The figure shows three views and two pictorial views of one solid part (mm, origin at its lowest corner). Answer the questions. Coordinates: 2 decimals unless noted, no trailing zeros. Loops run counter-clockwise (first coordinate to the right, second up) from the corner with the lowest first, then second, coordinate; pieces in that order, holes last. Notation, with made-up numbers: M -20,0 L -5,0 A26 cw -5,27 Z; hole C 35.25,-27 d11. An arc over 180 degrees is marked long. Write each question's results on one line, items separated by ' | '.
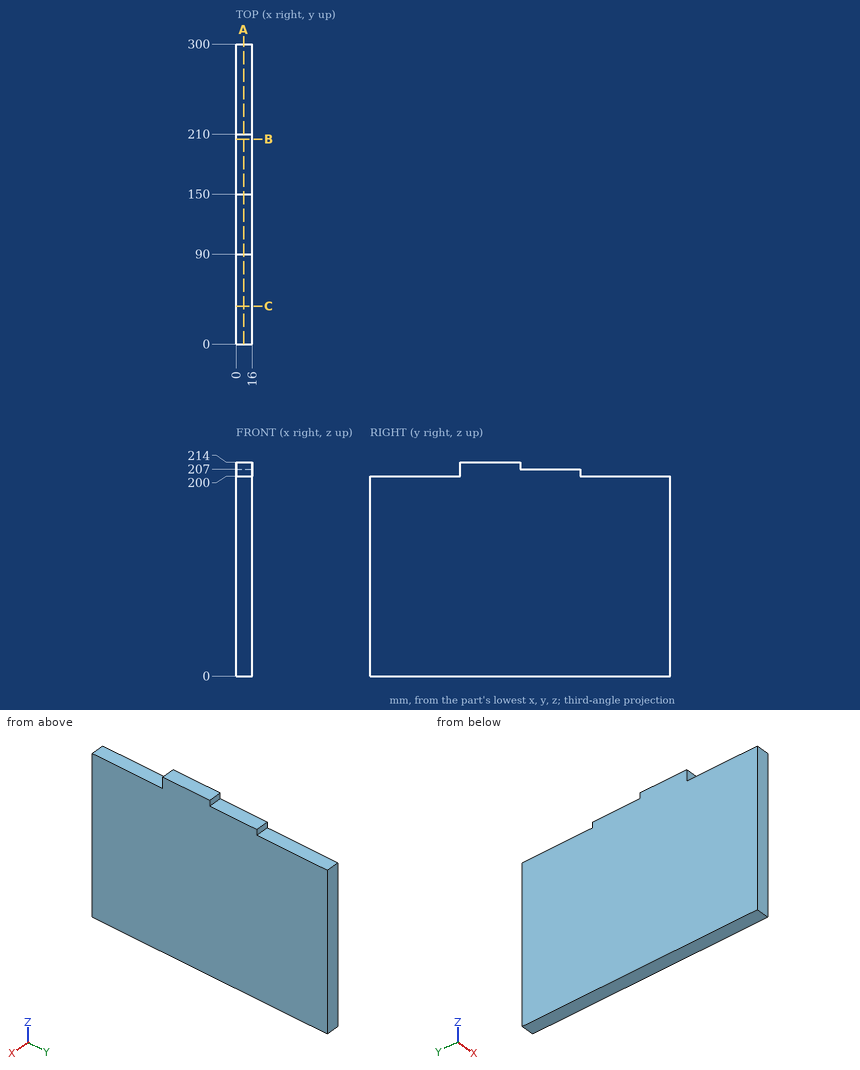
1) Straight lines are drawn through the part: probe 1 along Z at (x, y) = (7, 80.5); probe 2 along Z at (x, y) = (3.75, 168). For each, find the intervals that lie inside material, in ascending order. Write a range as [from, to].
Check result:
probe 1: [0, 200] | probe 2: [0, 207]
2) Find section C-C, the plane y = 38. Give the vertices of the cut face in (x, z), and give its area (3 significant figures).
Check result:
outline: M 0,0 L 16,0 L 16,200 L 0,200 Z | area: 3,200 mm^2
3) Find section B-B, the plane y = 205. Give the vertices of the cut face in (x, z), and give its area (3 significant figures).
Check result:
outline: M 0,0 L 16,0 L 16,207 L 0,207 Z | area: 3,310 mm^2
4) Given pin 1 Ø8 at (x, y) = (8.5, 189) entering from +Z; pin 2 Ø3.5 at (x, z) = (10, 204) entering from +Y; pin 3 Ø2 at (x, z) = (11.5, 210.5) entering from +Y, each flat-ended and moving along its own axis, determine where each tip first touches the part or whether it passes through.
Check result:
pin 1: z = 207 | pin 2: y = 210 | pin 3: y = 150
5) Find section A-A, the plane x = 7.5. Give the vertices of the cut face in (y, z), and give its area (3 significant figures).
Check result:
outline: M 0,0 L 300,0 L 300,200 L 210,200 L 210,207 L 150,207 L 150,214 L 90,214 L 90,200 L 0,200 Z | area: 61,300 mm^2
